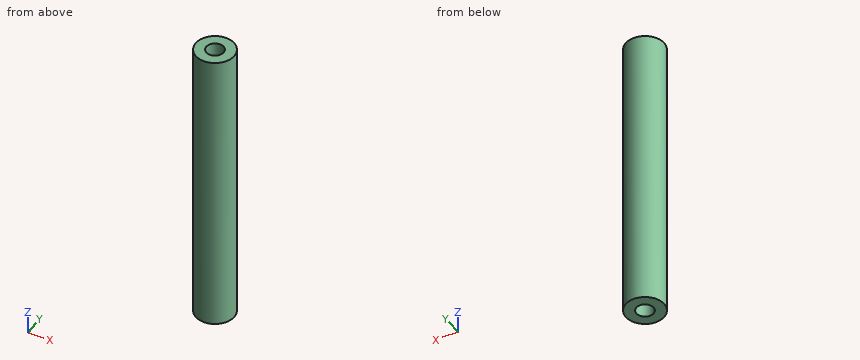
```python
from build123d import *

# Parameters (mm, degrees)
SKETCH1_R                 = 3
BOSS_EXTRUDE1_DEPTH       = 45.28
F_6_32_TAPPED_HOLE1_D     = 2.7051
F_6_32_TAPPED_HOLE1_DEPTH = 10
F_6_32_TAPPED_HOLE1_TIP   = 0.81269403
F_6_32_TAPPED_HOLE2_D     = 2.7051
F_6_32_TAPPED_HOLE2_DEPTH = 10
F_6_32_TAPPED_HOLE2_TIP   = 0.81269403


with BuildPart() as part:
    # Sketch1 → Boss-Extrude1 (new body)
    with BuildSketch(Plane.XY):
        Circle(SKETCH1_R)
    extrude(amount=BOSS_EXTRUDE1_DEPTH)

    # #6-32 Tapped Hole1
    with Locations(Plane.XY.offset(45.28)):
        with Locations((0, 0)):
            Hole(F_6_32_TAPPED_HOLE1_D / 2, depth=F_6_32_TAPPED_HOLE1_DEPTH)
            with Locations((0, 0, -(F_6_32_TAPPED_HOLE1_DEPTH + F_6_32_TAPPED_HOLE1_TIP / 2))):  # 118° drill point
                Cone(0, F_6_32_TAPPED_HOLE1_D / 2, F_6_32_TAPPED_HOLE1_TIP, mode=Mode.SUBTRACT)

    # #6-32 Tapped Hole2
    with Locations(Plane(origin=(0, 0, 0), x_dir=(-1, 0, 0), z_dir=(0, 0, -1))):
        with Locations((0, 0)):
            Hole(F_6_32_TAPPED_HOLE2_D / 2, depth=F_6_32_TAPPED_HOLE2_DEPTH)
            with Locations((0, 0, -(F_6_32_TAPPED_HOLE2_DEPTH + F_6_32_TAPPED_HOLE2_TIP / 2))):  # 118° drill point
                Cone(0, F_6_32_TAPPED_HOLE2_D / 2, F_6_32_TAPPED_HOLE2_TIP, mode=Mode.SUBTRACT)


solid = part.part
```
Part model, mm, in its own coordinate system. Round coordinates to 2 decimals unless told otherwise and drop trailing zeros. Order: outer loops, then holes, each group sorted by start corner. A loop starts at its lowest first (then second) coordinate and runs counter-clockwise, first axis right, second up. Notation, with made-up numbers: M 75,-18.75 L 124,-18.75 A22 cw 124,-4.75 Z; hole C -10.5,81 d7. An arc over 180 degrees is marked long. Put each result on its own line as item: value. Start each with the question number.
1. Slice it at D-D on x = -2.6. List the corners of the cut face in (y, z).
2. Drop flat-ended pins along their axis: pin 1 (2.5 mm diameter, centred on x = 0, y = 0, fed in from -Z); pin 2 (1 mm diameter, centred on x = -0.5, y = -1, fed in from +Z). Give the stop position or say it passes through.
3. Slice it at C-C on x = 1.85. List the corners of the cut face in (y, z), then the cut area to 3 significant figures.
4. Slice it at B-B on z = 40.5. List the corners of the cut face in (x, y), then the cut area to 3 significant figures.
5. Slice it at A-A on z = 23.5. List the corners of the cut face in (x, y), then the cut area to 3 significant figures.
6. Drill centre lines: probe 1 along Y at (x, z) = (0, 2.5); probe 2 along Z at (x, y) = (0.8, -0.1); probe 3 along X at (y, z) = (-0.25, 14.5). Where is each one in solid material? Low to high. Write a range as [from, to].
Findings:
1. outline: M -1.5,0 L 1.5,0 L 1.5,45.28 L -1.5,45.28 Z
2. pin 1: z = 10.06
2. pin 2: z = 45.28
3. outline: M -2.36,0 L 2.36,0 L 2.36,45.28 L -2.36,45.28 Z
3. area: 214 mm2
4. outline: C 0,0 d6; hole C 0,0 d2.71
4. area: 22.5 mm2
5. outline: C 0,0 d6
5. area: 28.3 mm2
6. probe 1: [-3, -1.35], [1.35, 3]
6. probe 2: [10.33, 34.95]
6. probe 3: [-2.99, 2.99]
